from build123d import *

# Parameters (mm, degrees)
SKETCH1_W           = 50.8
SKETCH1_H           = 50.8
BOSS_EXTRUDE1_DEPTH = 1.5875
SKETCH3_R           = 1.5875
BOSS_EXTRUDE2_DEPTH = 7.62
SKETCH4_R           = 2.54
SKETCH4_R_2         = 1.27
CUT_EXTRUDE1_DEPTH  = 42.77991174


with BuildPart() as part:
    # Sketch1 → Boss-Extrude1 (new, symmetric)
    with BuildSketch(Plane(origin=(0, 0, 0), x_dir=(1, 0, 0), z_dir=(0, 1, 0))):
        Rectangle(SKETCH1_W, SKETCH1_H)
    extrude(amount=BOSS_EXTRUDE1_DEPTH, both=True)

    # Sketch3 → Boss-Extrude2 (add)
    with BuildSketch(Plane(origin=(25.4, 0, 0), x_dir=(0, 0, -1), z_dir=(1, 0, 0))):
        with Locations(Location((0, 0, 0), (0, 0, 270))):
            Circle(SKETCH3_R)
    boss_extrude2 = extrude(amount=BOSS_EXTRUDE2_DEPTH)

    # Mirror1: Boss-Extrude2 across plane
    add(boss_extrude2.mirror(Plane(origin=(0, 0, 0), x_dir=(0, 0, 1), z_dir=(1, 0, 0))))

    # Sketch4 → Cut-Extrude1 (cut, through all)
    with BuildSketch(Plane(origin=(0, 1.5875, 0), x_dir=(1, 0, 0), z_dir=(0, 1, 0))):
        with Locations(Location((0, 0, 0), (0, 0, 270))):
            Circle(SKETCH4_R)
        with Locations(Location((-16.51, 16.51, 0), (0, 0, 270))):
            Circle(SKETCH4_R)
        with Locations(Location((16.51, 16.51, 0), (0, 0, 270))):
            Circle(SKETCH4_R)
        with Locations(Location((16.51, -16.51, 0), (0, 0, 270))):
            Circle(SKETCH4_R)
        with Locations(Location((-16.51, -16.51, 0), (0, 0, 270))):
            Circle(SKETCH4_R)
        with Locations(Location((-16.51, 7.62, 0), (0, 0, 270))):
            Circle(SKETCH4_R_2)
        with Locations(Location((-7.62, 16.51, 0), (0, 0, 270))):
            Circle(SKETCH4_R_2)
        with Locations(Location((7.62, 16.51, 0), (0, 0, 270))):
            Circle(SKETCH4_R_2)
        with Locations(Location((-16.51, -7.62, 0), (0, 0, 270))):
            Circle(SKETCH4_R_2)
        with Locations(Location((7.62, -16.51, 0), (0, 0, 90))):
            Circle(SKETCH4_R_2)
        with Locations(Location((-7.62, -16.51, 0), (0, 0, 90))):
            Circle(SKETCH4_R_2)
        with Locations(Location((16.51, -7.62, 0), (0, 0, 90))):
            Circle(SKETCH4_R_2)
        with Locations(Location((16.51, 7.62, 0), (0, 0, 90))):
            Circle(SKETCH4_R_2)
        with Locations(Location((5.578227154, 8.89, 0), (0, 0, 270))):
            Circle(SKETCH4_R_2)
        with Locations(Location((-5.578227154, 8.89, 0), (0, 0, 270))):
            Circle(SKETCH4_R_2)
        with Locations(Location((8.89, -5.578227154, 0), (0, 0, 270))):
            Circle(SKETCH4_R_2)
        with Locations(Location((8.89, 5.578227154, 0), (0, 0, 270))):
            Circle(SKETCH4_R_2)
        with Locations(Location((-5.578227154, -8.89, 0), (0, 0, 270))):
            Circle(SKETCH4_R_2)
        with Locations(Location((5.578227154, -8.89, 0), (0, 0, 270))):
            Circle(SKETCH4_R_2)
        with Locations(Location((-8.89, 5.578227154, 0), (0, 0, 270))):
            Circle(SKETCH4_R_2)
        with Locations(Location((-8.89, -5.578227154, 0), (0, 0, 270))):
            Circle(SKETCH4_R_2)
    extrude(amount=-CUT_EXTRUDE1_DEPTH, mode=Mode.SUBTRACT)


solid = part.part
Build history of the part. All positions in model axes, mm. A direction names the side the tool comes from. Coordinates: 2 decimals unless noted, no trailing zeros. Write each loop counter-clockwise with the first axis right and the second up, starting at its lowest first coordinate (ties: lowest second). Pieces come first, ordered by that corner, then holes.
(1) Cut at B-B on x = 16.51. List the corners of the cut face in (y, z).
(2) Cut at A-A on z = 16.51. List the corners of the cut face in (x, y).
(3) Mould opens along X. For faces 3 (the cylindrical face through (-17.483, 0.022, -14.164)), 4 (the flat face through (0, 0, -25.4)), 5 (the flat face through (-25.4, 0, -13)) say: pulls with the +X half, pulls with the -X half, needs draft (parallel to the pull), parting line crosses it, or undercut.
(4) Cut at C-C on y = -0.9. State how many separate pieces and enclosed holes the cut face has, and give its area (3 significant figures).
(5) Cut at D-D on z = 5. List the corners of the cut face in (x, y), and give its area (3 significant figures).
(6) Pin check, flat tips, straight feed: pin 1 Ø1 at (y, z) = (0.5, 11) entering from -X; pin 2 Ø3.5 at (x, z) = (-8.89, -5.58) entering from -Y; pin 3 Ø1.6 at (y, z) = (-0.5, 16) entering from +X. Stop position of each tip, or through.
(7) 3-axis set-ups, long thin cutter, end or side, ignore diameter. For faces 1 (the cylindrical face through (-29.157, 1.26, 0.966)), 2 (the cylindrical face through (5.092, 0.022, 10.063)): which of +Z, -Z, +X, -X, +Y, -Y reach the whole face in a straight line?
(8) Drill centre lines: line 1 (X direction, y = 0.95, z = 16.51); line 2 (X direction, y = 0.95, z = 7.5); line 3 (X direction, y = -0.2, z = 5.5). Where is each one in solid material? Low to high.
Working result:
1. outline: (-1.59, -25.4) - (1.59, -25.4) - (1.59, -19.05) - (-1.59, -19.05) - close; (-1.59, -13.97) - (1.59, -13.97) - (1.59, -8.89) - (-1.59, -8.89) - close; (-1.59, -6.35) - (1.59, -6.35) - (1.59, 6.35) - (-1.59, 6.35) - close; (-1.59, 8.89) - (1.59, 8.89) - (1.59, 13.97) - (-1.59, 13.97) - close; (-1.59, 19.05) - (1.59, 19.05) - (1.59, 25.4) - (-1.59, 25.4) - close
2. outline: (-25.4, -1.59) - (-19.05, -1.59) - (-19.05, 1.59) - (-25.4, 1.59) - close; (-13.97, -1.59) - (-8.89, -1.59) - (-8.89, 1.59) - (-13.97, 1.59) - close; (-6.35, -1.59) - (6.35, -1.59) - (6.35, 1.59) - (-6.35, 1.59) - close; (8.89, -1.59) - (13.97, -1.59) - (13.97, 1.59) - (8.89, 1.59) - close; (19.05, -1.59) - (25.4, -1.59) - (25.4, 1.59) - (19.05, 1.59) - close
3. face 3: undercut
3. face 4: needs draft
3. face 5: pulls with the -X half
4. separate pieces: 1
4. enclosed holes: 21
4. area: 2,440 mm2
5. outline: (-25.4, -1.59) - (-10.02, -1.59) - (-10.02, 1.59) - (-25.4, 1.59) - close; (-7.76, -1.59) - (7.76, -1.59) - (7.76, 1.59) - (-7.76, 1.59) - close; (10.02, -1.59) - (25.4, -1.59) - (25.4, 1.59) - (10.02, 1.59) - close
5. area: 147 mm2
6. pin 1: stops at x = -25.4
6. pin 2: stops at y = -1.59
6. pin 3: stops at x = 25.4
7. face 1: -X
7. face 2: +Y, -Y
8. line 1: x = -25.4 to -19.05, -13.97 to -8.89, -6.35 to 6.35, 8.89 to 13.97, 19.05 to 25.4
8. line 2: x = -25.4 to -17.77, -15.25 to 15.25, 17.77 to 25.4
8. line 3: x = -25.4 to -10.16, -7.62 to 7.62, 10.16 to 25.4
